from build123d import *

# Parameters (mm, degrees)
SKETCH_1_W          = 129.17
SKETCH_1_H          = 116.67
SKETCH_1_W_2        = 88.65
SKETCH_1_H_2        = 76.19
EXTRUDE_1_DEPTH     = 6
SKETCH_2_R          = 1.55
CUT_EXTRUDE_1_DEPTH = 115.383560689


with BuildPart() as part:
    # Эскиз1 → Бобышка-Вытянуть1 (new body)
    with BuildSketch(Plane.XY):
        with Locations((7.986729107, -29.874654179)):
            Rectangle(SKETCH_1_W, SKETCH_1_H)
        with Locations((7.986729107, -29.874654179)):
            Rectangle(SKETCH_1_W_2, SKETCH_1_H_2, mode=Mode.SUBTRACT)
    extrude(amount=EXTRUDE_1_DEPTH)

    # Эскиз2 → Вырез-Вытянуть1 (cut, through all)
    with BuildSketch(Plane(origin=(0, 0, 0), x_dir=(-1, 0, 0), z_dir=(0, 0, -1))):
        with Locations((46.464144791, -15.068841065)):
            Circle(SKETCH_2_R)
        with Locations((46.464144791, -44.679267292)):
            Circle(SKETCH_2_R)
        with Locations((13.069084007, -78.074328076)):
            Circle(SKETCH_2_R)
        with Locations((-29.04134222, -78.074328076)):
            Circle(SKETCH_2_R)
        with Locations((-62.436403004, -44.679267292)):
            Circle(SKETCH_2_R)
        with Locations((-62.436403004, -15.068841065)):
            Circle(SKETCH_2_R)
        with Locations((-29.04134222, 18.326219719)):
            Circle(SKETCH_2_R)
        with Locations((13.069084007, 18.326219719)):
            Circle(SKETCH_2_R)
    extrude(amount=-CUT_EXTRUDE_1_DEPTH, mode=Mode.SUBTRACT)


solid = part.part
Could you check a few things on this model? Use its own coordinates, in mm. A direction names the side the tool comes from. Give positions to 0.01 mm unless a question says otherwise; leave off trailing zeros. Order: outer loops, then holes, each group sorted by start corner. A loop starts at its lowest first (then second) coordinate and runs counter-clockwise, first axis right, second up. Notation, with made-up numbers: (73.25, 58.5) - (100.25, 58.5) arc R11 cw to (100.25, 72.5) - close; hole circle Ø11 at (46, 14). An arc over 180 degrees is marked (long way). One line per question, with ' | ' between items. Start each with the question number.
Item 1: Thinking about a two-plate mould opening in X: for faces 1 (the flat face through (-36.338, -30, 3)), 2 (the flat face through (-56.598, -31, 3)), 3 (the flat face through (52.312, -30, 3)), 4 (the flat face through (7, 10, 0)), which applies, pulls with the +X half, pulls with the -X half, needs draft (parallel to the pull), parting line crosses it, or undercut?
Item 2: I want a section at B-B on y = -51.5. Write out the boundary of the cut face in (x, z).
Item 3: I want a section at C-C on z = 1.7. Give the number of separate pieces and of enclosed holes in the cut face, then the cut area to 3 significant figures.
Item 4: For faces 5 (the flat face through (7, -88.21, 3)), 6 (the flat face through (7, -67.97, 3)), which set-ups out of +Z, -Z, +X, -X, +Y, -Y let a thin tool reach every point of the face, with its end or its side?
Item 5: I want a section at A-A on x = 48. Write out the boundary of the cut face in (y, z).
Item 6: I need wall thicknesses on probe 1 along X at (y, z) = (-15, 2.8); probe 2 along X at (y, z) = (-29, 5.75); probe 3 along Y at (x, z) = (34, 1.95). Which ranges of each line are inside material? Lowest first, please. Write a range as [from, to].
Verdict:
1) face 1: undercut | face 2: pulls with the -X half | face 3: undercut | face 4: needs draft
2) outline: (-56.6, 0) - (-36.34, 0) - (-36.34, 6) - (-56.6, 6) - close; (52.31, 0) - (72.57, 0) - (72.57, 6) - (52.31, 6) - close
3) separate pieces: 1 | enclosed holes: 9 | area: 8,260 mm^2
4) face 5: +Z, -Z, +X, -X, -Y | face 6: +Z, -Z
5) outline: (-88.21, 0) - (-67.97, 0) - (-67.97, 6) - (-88.21, 6) - close; (8.22, 0) - (28.46, 0) - (28.46, 6) - (8.22, 6) - close
6) probe 1: [-56.6, -48.01], [-44.92, -36.34], [52.31, 60.89], [63.98, 72.57] | probe 2: [-56.6, -36.34], [52.31, 72.57] | probe 3: [-88.21, -67.97], [8.22, 28.46]
